from build123d import *

# Parameters (mm, degrees)
SKETCH1_R                  = 17
BOSS_EXTRUDE1_DEPTH        = 10
F_3_7_3_7_DIAMETER_HOLE1_D = 3.7
M5_TAPPED_HOLE1_D          = 4.2
F_12_0_12_DIAMETER_HOLE1_D = 8
CUT_EXTRUDE3_DEPTH         = 5
CIRPATTERN1_COUNT          = 4
SKETCH21_R                 = 3.25
CUT_EXTRUDE4_DEPTH         = 27.038433302
CUT_EXTRUDE5_DEPTH         = 27.038433302


with BuildPart() as part:
    # Sketch1 → Boss-Extrude1 (new body)
    with BuildSketch(Plane(origin=(0, 0, 0), x_dir=(1, 0, 0), z_dir=(0, 1, 0))):
        with Locations(Location((0, 0, 0), (0, 0, 270))):
            Circle(SKETCH1_R)
    extrude(amount=BOSS_EXTRUDE1_DEPTH)

    # Ø3.7 (3.7) Diameter Hole1 (through all)
    with Locations(Plane(origin=(0, 10, 0), x_dir=(1, 0, 0), z_dir=(0, 1, 0))):
        with Locations((-12.5, 0), (12.5, 0)):
            Hole(F_3_7_3_7_DIAMETER_HOLE1_D / 2)

    # M5 Tapped Hole1 (through all)
    with Locations(Plane(origin=(0, 10, 0), x_dir=(1, 0, 0), z_dir=(0, 1, 0))):
        with Locations((0, 8), (0, -8)):
            Hole(M5_TAPPED_HOLE1_D / 2)

    # Ø12.0 (12) Diameter Hole1 (through all)
    with Locations(Plane(origin=(0, 10, 0), x_dir=(1, 0, 0), z_dir=(0, 1, 0))):
        with Locations((0, 0)):
            Hole(F_12_0_12_DIAMETER_HOLE1_D / 2)

    # Sketch16 → Cut-Extrude3 (cut)
    with BuildSketch(Plane(origin=(0, 10, 0), x_dir=(1, 0, 0), z_dir=(0, 1, 0))):
        with BuildLine():
            Line((-16.487793391, 4.015586089), (-18.960782116, 4.015586089))
            Line((-18.960782116, 4.015586089), (-18.960782116, -4.01131039))
            Line((-18.960782116, -4.01131039), (-16.488958096, -4.01131039))
            ThreePointArc((-16.488958096, -4.01131039), (-15.936832629, -3.116268297), (-14.889208553, -3.208065225))
            ThreePointArc((-14.889208553, -3.208065225), (-8.500000472, -0.001943416), (-14.886090124, 3.210385323))
            ThreePointArc((-14.886090124, 3.210385323), (-15.935159239, 3.119232137), (-16.487793391, 4.015586089))
        make_face()
        with BuildLine():
            Line((16.487793391, -4.015586089), (18.960782116, -4.015586089))
            Line((18.960782116, -4.015586089), (18.960782116, 4.01131039))
            Line((18.960782116, 4.01131039), (16.488958096, 4.01131039))
            ThreePointArc((16.488958096, 4.01131039), (15.936832629, 3.116268297), (14.889208553, 3.208065225))
            ThreePointArc((14.889208553, 3.208065225), (8.500000472, 0.001943416), (14.886090124, -3.210385323))
            ThreePointArc((14.886090124, -3.210385323), (15.935159239, -3.119232137), (16.487793391, -4.015586089))
        make_face()
    extrude(amount=-CUT_EXTRUDE3_DEPTH, mode=Mode.SUBTRACT)

    # Sketch18 → M2 Tapped Hole1 (revolve, cut)
    with BuildSketch(Plane(origin=(15.40723238, 5, 7.18451045), x_dir=(0.42261826174070016, 0, -0.9063077870366497), z_dir=(0, 1, 0))):
        Polygon((0, 0), (0, 4.480688495), (0.8, 4), (0.8, 0), align=None)
    m2_tapped_hole1 = revolve(axis=Axis((21.162286827, 5, 9.868136412), (-0.9063077870366497, 0, -0.42261826174070016)), mode=Mode.SUBTRACT)

    # CirPattern1: M2 Tapped Hole1 ×4 about axis
    cirpattern1_axis = Axis((0, 0, 0), (0, 1, 0))
    for i in range(1, CIRPATTERN1_COUNT):
        add(m2_tapped_hole1.rotate(cirpattern1_axis, i * 360 / CIRPATTERN1_COUNT), mode=Mode.SUBTRACT)

    # Sketch21 → Cut-Extrude4 (cut, through all)
    with BuildSketch(Plane(origin=(0, 10, 0), x_dir=(1, 0, 0), z_dir=(0, 1, 0))):
        with Locations(Location((-8, 8, 0), (0, 0, 270))):
            Circle(SKETCH21_R)
        with Locations(Location((8, 8, 0), (0, 0, 270))):
            Circle(SKETCH21_R)
        with Locations(Location((8, -8, 0), (0, 0, 270))):
            Circle(SKETCH21_R)
        with Locations(Location((-8, -8, 0), (0, 0, 270))):
            Circle(SKETCH21_R)
    extrude(amount=-CUT_EXTRUDE4_DEPTH, mode=Mode.SUBTRACT)

    # Sketch14 → Cut-Extrude5 (cut, through all)
    with BuildSketch(Plane(origin=(0, 10, 0), x_dir=(1, 0, 0), z_dir=(0, 1, 0))):
        with BuildLine():
            Line((-1.459621356, 16.913091325), (-1.166781334, 18.506531105))
            Line((-1.166781334, 18.506531105), (1.608035184, 18.356142043))
            Line((1.608035184, 18.356142043), (1.452856339, 16.913870267))
            ThreePointArc((1.452856339, 16.913870267), (0.984569232, 16.476462251), (1.174122642, 15.864344539))
            ThreePointArc((1.174122642, 15.864344539), (0.000614681, 12.700000105), (-1.175054186, 15.86354232))
            ThreePointArc((-1.175054186, 15.86354232), (-0.986764651, 16.477946041), (-1.459621356, 16.913091325))
        make_face()
        with BuildLine():
            Line((1.459621356, -16.913091325), (1.166781334, -18.506531105))
            Line((1.166781334, -18.506531105), (-1.608035184, -18.356142043))
            Line((-1.608035184, -18.356142043), (-1.452856339, -16.913870267))
            ThreePointArc((-1.452856339, -16.913870267), (-0.984569232, -16.476462251), (-1.174122642, -15.864344539))
            ThreePointArc((-1.174122642, -15.864344539), (-0.000614681, -12.700000105), (1.175054186, -15.86354232))
            ThreePointArc((1.175054186, -15.86354232), (0.986764651, -16.477946041), (1.459621356, -16.913091325))
        make_face()
    extrude(amount=-CUT_EXTRUDE5_DEPTH, mode=Mode.SUBTRACT)


solid = part.part
Part model, mm, in its own coordinate system. A direction names the side the tool comes from. Coordinates: 2 decimals unless noted, no trailing zeros. Order: outer loops, then holes, each group sorted by start corner. A loop starts at its lowest first (then second) coordinate and runs counter-clockwise, first axis right, second up.
(1) Pin check, flat tips, straight feed: pin 1 Ø4 at (x, z) = (14, 0.5) entering from +Y; pin 2 Ø8.5 at (x, z) = (-8, -8) entering from +Y; pin 3 Ø2 at (x, y) = (-4, 8.5) entering from +Z. Stop position of each tip, or through.
Check sheet entries:
pin 1: stops at y = 5
pin 2: stops at y = 10
pin 3: stops at z = 16.73
(2) Slice it at A-A, the plane x = 0. Write the cut outline in (y, z), and give its area (3 significant figures).
Check sheet entries:
outline: (0, -12.7) - (10, -12.7) - (10, -10.1) - (0, -10.1) - close; (0, -5.9) - (10, -5.9) - (10, -4) - (0, -4) - close; (0, 4) - (10, 4) - (10, 5.9) - (0, 5.9) - close; (0, 10.1) - (10, 10.1) - (10, 12.7) - (0, 12.7) - close
area: 90.0 mm2
(3) Pull direction Z, two halves, no side cores. Call faces 1 (the face through (10.79, 2.47, 0.71)), 2 (the face through (17, 4, 0)), 3 (the face through (4, 10, -4)): pulls with the +Z half, pulls with the -Z half, needs draft (parallel to the pull), parting line crosses it, or undercut.
Check sheet entries:
face 1: undercut
face 2: parting line crosses it
face 3: needs draft
(4) Slice it at B-B, the plane z = -1. Write the cut outline in (x, y).
Check sheet entries:
outline: (-16.97, 0) - (-14.06, 0) - (-14.06, 5) - (-16.97, 5) - close; (-10.94, 0) - (-3.87, 0) - (-3.87, 10) - (-8.63, 10) - (-8.63, 5) - (-10.94, 5) - close; (3.87, 0) - (10.94, 0) - (10.94, 5) - (8.63, 5) - (8.63, 10) - (3.87, 10) - close; (14.06, 0) - (16.97, 0) - (16.97, 5) - (14.06, 5) - close
(5) Probe L1, parallel to Z at x = 0, y = 3.75; L2, parallel to Z at x = -5, y = 3.25; L3, parallel to Z at x = -11, y = 3.75. List the from-to ranges inside material, lowest first.
Check sheet entries:
L1: z = -12.7 to -10.1, -5.9 to -4, 4 to 5.9, 10.1 to 12.7
L2: z = -16.25 to -9.25, -6.75 to 6.75, 9.25 to 16.25
L3: z = -12.96 to -9.25, -6.75 to -1.08, 1.08 to 6.75, 9.25 to 12.96
(6) Slice it at C-C, the plane y = 8.5. State how many separate pieces and enclosed holes the cut face has, and give its area (3 significant figures).
Check sheet entries:
separate pieces: 1
enclosed holes: 7
area: 561 mm2
(7) Tool access for faces 4 (the face through (5.419, 4.906, -11.379)), 5 (the face through (0.984, 5.07, 16.469)), 6 (the face through (-17, 4, 0)), 7 (the face through (-8.5, 7.5, 0.1)): list every direction of +Z, -Z, +X, -X, +Y, -Y with a clear straight run to the whole face (end or side of a thin tool).
Check sheet entries:
face 4: none
face 5: +Y, -Y
face 6: -X, +Y, -Y
face 7: +Y
